Here's how the part is built. I have some questions about the finished solid (model axes, mm). Give positions to 0.01 mm unless a question says otherwise; leave off trailing zeros. Loops run counter-clockwise (first coordinate to the right, second up) from the corner with the lowest first, then second, coordinate; pieces in that order, holes last.
Q1. I need wall thicknesses on probe 1 along Z at (x, y) = (132.5, -1.3); probe 2 along X at (y, z) = (-1.9, 71); probe 3 along Z at (x, y) = (-40.5, -1.3). Which ranges of each line are inside material? Lowest first, please.
Q2. I'm going to push flat-ended pins straight in: P1, Ø2.5, axis at x = -75, z = 87.5, coming from the +Y side; P2, Ø1, axis at x = 7, y = -0.5, coming from the -Z side. Where does each tip first touch, or does it pass through?
Q3. Suppose I cut it at B-B (y = -0.3). Count the separate pieces of the cut face and the enclosed holes in it, and give its area (3 significant figures).
Q4. Suppose I cut it at A-A (x = -43). List the corners of the cut face in (y, z) for me, and give its area (3 significant figures).
```python
from build123d import *

# Parameters (mm, degrees)
BOSS_EXTRUDE1_DEPTH  = 2
SKETCH8_R            = 2.15
CUT_EXTRUDE11_DEPTH  = 185.011548551
CUT_EXTRUDE12_DEPTH  = 185.011548551
FILLET1_R            = 7
SKETCH11_R           = 6.5
CUT_EXTRUDE14_DEPTH  = 185.011548551
SKETCH10_R           = 2.15
CUT_EXTRUDE13_DEPTH  = 185.011548551
LPATTERN1_COUNT      = 8
LPATTERN1_PITCH      = 25
LPATTERN1_COUNT_DIR2 = 11
LPATTERN1_PITCH_DIR2 = 25
SKETCH18_R           = 1.65
CUT_EXTRUDE21_DEPTH  = 185.011548551
CUT_EXTRUDE22_DEPTH  = 10
SKETCH20_R           = 2.15
BOSS_EXTRUDE2_DEPTH  = 2
SKETCH23_R           = 3.5
CUT_EXTRUDE25_DEPTH  = 10


with BuildPart() as part:
    # Sketch1 → Boss-Extrude1 (new body)
    with BuildSketch(Plane(origin=(0, 0, 0), x_dir=(1, 0, 0), z_dir=(0, 1, 0))):
        with BuildLine():
            Line((117.5, -110), (-117.5, -110))
            ThreePointArc((-117.5, -110), (-138.713203436, -101.213203436), (-147.5, -80))
            Line((-147.5, -80), (-147.5, 80))
            ThreePointArc((-147.5, 80), (-138.713203436, 101.213203436), (-117.5, 110))
            Line((-117.5, 110), (117.5, 110))
            ThreePointArc((117.5, 110), (138.713203436, 101.213203436), (147.5, 80))
            Line((147.5, 80), (147.5, -80))
            ThreePointArc((147.5, -80), (138.713203436, -101.213203436), (117.5, -110))
        make_face()
    extrude(amount=-BOSS_EXTRUDE1_DEPTH)

    # Sketch8 → Cut-Extrude11 (cut, through all)
    with BuildSketch(Plane(origin=(0, 0, 0), x_dir=(1, 0, 0), z_dir=(0, 1, 0))):
        with Locations(Location((-132.5, 90, 0), (0, 0, 270))):
            Circle(SKETCH8_R)
        with Locations(Location((132.5, 90, 0), (0, 0, 270))):
            Circle(SKETCH8_R)
        with Locations(Location((-132.5, -90, 0), (0, 0, 270))):
            Circle(SKETCH8_R)
        with Locations(Location((132.5, -90, 0), (0, 0, 270))):
            Circle(SKETCH8_R)
    extrude(amount=-CUT_EXTRUDE11_DEPTH, mode=Mode.SUBTRACT)

    # Sketch9 → Cut-Extrude12 (cut, through all)
    with BuildSketch(Plane(origin=(0, 0, 0), x_dir=(1, 0, 0), z_dir=(0, 1, 0))):
        Polygon((-75, -110), (-67, -102), (67, -102), (75, -110), align=None)
    cut_extrude12 = extrude(amount=-CUT_EXTRUDE12_DEPTH, mode=Mode.SUBTRACT)

    # Mirror2: Cut-Extrude12 across plane
    add(cut_extrude12.mirror(Plane.XY), mode=Mode.SUBTRACT)

    # Fillet1
    fillet1_edges = [part.edges().sort_by_distance(p)[0] for p in [
        (75, -1, 110),
        (-75, -1, 110),
        (-67, -1, 102),
        (67, -1, 102),
        (-75, -1, -110),
        (75, -1, -110),
        (67, -1, -102),
        (-67, -1, -102),
    ]]
    fillet(fillet1_edges, radius=FILLET1_R)

    # Sketch11 → Cut-Extrude14 (cut, through all)
    with BuildSketch(Plane(origin=(0, 0, 0), x_dir=(1, 0, 0), z_dir=(0, 1, 0))):
        with Locations(Location((0, -37.5, 0), (0, 0, 270))):
            Circle(SKETCH11_R)
    extrude(amount=-CUT_EXTRUDE14_DEPTH, mode=Mode.SUBTRACT)

    # Sketch10 → Cut-Extrude13 (cut, through all)
    with BuildSketch(Plane(origin=(0, 0, 0), x_dir=(1, 0, 0), z_dir=(0, 1, 0))):
        with Locations(Location((-125, 87.5, 0), (0, 0, 270))):
            Circle(SKETCH10_R)
    cut_extrude13 = extrude(amount=-CUT_EXTRUDE13_DEPTH, mode=Mode.SUBTRACT)

    # LPattern1: Cut-Extrude13 8 × 11, 7 skipped
    with Locations(*[(j * LPATTERN1_PITCH_DIR2, 0, i * LPATTERN1_PITCH) for i in range(LPATTERN1_COUNT) for j in range(LPATTERN1_COUNT_DIR2) if (i, j) not in ((0, 0), (1, 4), (1, 5), (1, 6), (5, 5), (7, 4), (7, 5), (7, 6))]):
        add(cut_extrude13, mode=Mode.SUBTRACT)

    # Sketch18 → Cut-Extrude21 (cut, through all)
    with BuildSketch(Plane(origin=(0, 0, 0), x_dir=(1, 0, 0), z_dir=(0, 1, 0))):
        with Locations(Location((15, -72.5, 0), (0, 0, 270))):
            Circle(SKETCH18_R)
        with Locations(Location((-15, -72.5, 0), (0, 0, 270))):
            Circle(SKETCH18_R)
    extrude(amount=-CUT_EXTRUDE21_DEPTH, mode=Mode.SUBTRACT)

    # Sketch19 → Cut-Extrude22 (cut)
    with BuildSketch(Plane(origin=(0, 0, 0), x_dir=(1, 0, 0), z_dir=(0, 1, 0))):
        with BuildLine():
            Line((-11, -32.5), (11, -32.5))
            ThreePointArc((11, -32.5), (16, -37.5), (11, -42.5))
            Line((11, -42.5), (-11, -42.5))
            ThreePointArc((-11, -42.5), (-16, -37.5), (-11, -32.5))
        make_face()
    extrude(amount=-CUT_EXTRUDE22_DEPTH, mode=Mode.SUBTRACT)

    # Sketch20 → Boss-Extrude2 (add)
    with BuildSketch(Plane(origin=(0, 0, 0), x_dir=(1, 0, 0), z_dir=(0, 1, 0))):
        with Locations((125, 87.5)):
            Circle(SKETCH20_R)
        with Locations((125, -87.5)):
            Circle(SKETCH20_R)
        with Locations((-125, -87.5)):
            Circle(SKETCH20_R)
        with Locations((-125, 87.5)):
            Circle(SKETCH20_R)
    extrude(amount=-BOSS_EXTRUDE2_DEPTH)

    # Sketch23 → Cut-Extrude25 (cut)
    with BuildSketch(Plane(origin=(0, 0, 0), x_dir=(1, 0, 0), z_dir=(0, 1, 0))):
        with Locations(Location((0, 37.5, 0), (0, 0, 270))):
            Circle(SKETCH23_R)
    extrude(amount=-CUT_EXTRUDE25_DEPTH, mode=Mode.SUBTRACT)


solid = part.part
```
Solutions:
1. probe 1: z = -105.98 to -92.15, -87.85 to 87.85, 92.15 to 105.98
1. probe 2: x = -147.5 to -15.69, -14.31 to 14.31, 15.69 to 147.5
1. probe 3: z = -102 to 102
2. P1: passes through
2. P2: stops at z = -102
3. separate pieces: 1
3. enclosed holes: 84
3. area: 60,300 mm2
4. outline: (-2, -102) - (0, -102) - (0, 102) - (-2, 102) - close
4. area: 408 mm2
